Part print with two shaded views. Sizes in mm from the minimum x, y, z corner. A direction names the side the tool comes from. Round coordinates to 2 decimals unless told otherwise and drop trailing zeros. Loops run counter-clockwise (first coordinate to the right, second up) from the corner with the lowest first, then second, coordinate; pieces in that order, holes last. Notation, with made-up numbers: (34.25, 22) - (56.25, 22) arc R32 cw to (56.25, 53) - close; hole circle Ø11 at (-31, -27.5). An arc over 180 degrees is marked (long way). Put each result on its own line as item: value. Start each with the question number.
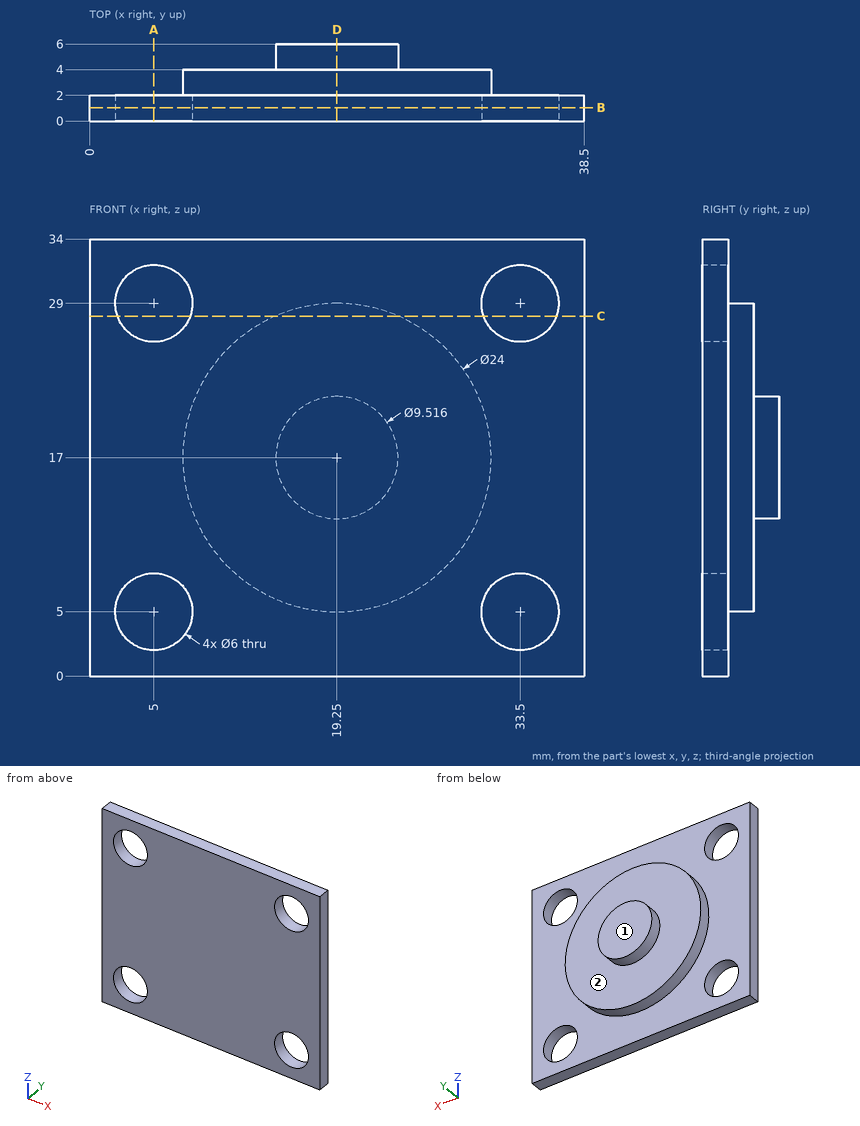
1) Slice it at D-D, the plane x = 19.25. Write the cut outline in (y, z), and give its area (3 significant figures).
2) Drill centre lines: line 1 (X direction, y = 0.8, z = 5); line 2 (Z direction, x = 34.5, y = 0.85); line 3 (X direction, y = 1.4, z = 3.5). Where is each one in solid material? Low to high. Write a range as [from, to].
3) Slice it at B-B, the plane y = 1.05. Write the cut outline in (x, z), and give its area (3 significant figures).
4) Drop a flat-ended pin along its axis: pin 1 Ø9.5 at (x, z) = (33.5, 29) entering from +Y. Give the stop position or say it passes through.
5) Which spindle directions (+Z, -Z, +X, -X, +Y, -Y) get a long thin tool onto all of the face, cutting with end or side? Do the marked faces 1 and 2. Say none if no direction does.
6) Slice it at A-A, the plane x = 5. Write the cut outline in (y, z), and give its area (3 significant figures).
7) Slice it at C-C, the plane z = 28. Write the cut outline in (x, y).
Taken from the geometry:
1. outline: (0, 0) - (2, 0) - (2, 5) - (4, 5) - (4, 12.24) - (6, 12.24) - (6, 21.76) - (4, 21.76) - (4, 29) - (2, 29) - (2, 34) - (0, 34) - close
1. area: 135 mm2
2. line 1: x = [0, 2], [8, 30.5], [36.5, 38.5]
2. line 2: z = [0, 2.17], [7.83, 26.17], [31.83, 34]
2. line 3: x = [0, 2.4], [7.6, 30.9], [36.1, 38.5]
3. outline: (0, 0) - (38.5, 0) - (38.5, 34) - (0, 34) - close; hole circle Ø6 at (5, 5); hole circle Ø6 at (5, 29); hole circle Ø6 at (33.5, 5); hole circle Ø6 at (33.5, 29)
3. area: 1,200 mm2
4. pin 1: stops at y = 2
5. face 1: +Z, -Z, +X, -X, +Y
5. face 2: +Y
6. outline: (0, 0) - (2, 0) - (2, 2) - (0, 2) - close; (0, 8) - (2, 8) - (2, 26) - (0, 26) - close; (0, 32) - (2, 32) - (2, 34) - (0, 34) - close
6. area: 44.0 mm2
7. outline: (0, 0) - (2.17, 0) - (2.17, 2) - (0, 2) - close; (7.83, 0) - (30.67, 0) - (30.67, 2) - (24.05, 2) - (24.05, 4) - (14.45, 4) - (14.45, 2) - (7.83, 2) - close; (36.33, 0) - (38.5, 0) - (38.5, 2) - (36.33, 2) - close
